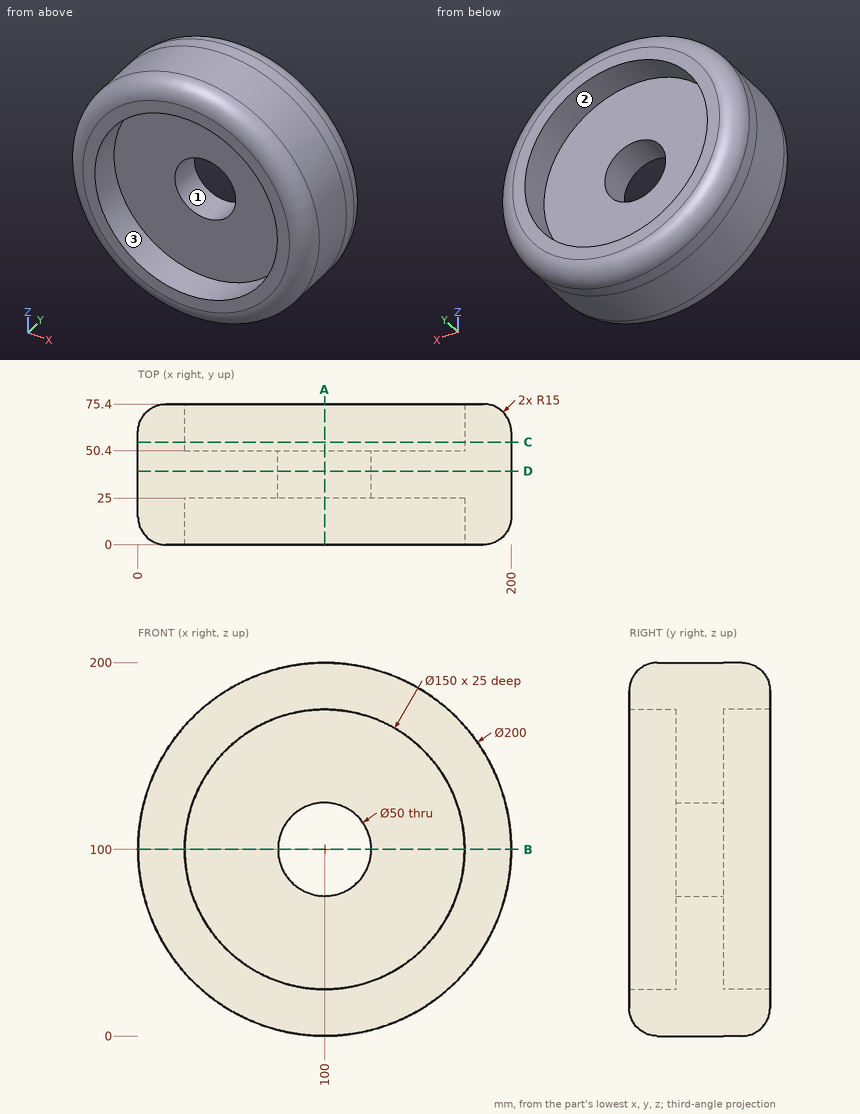
Here's the drawing with two shaded views (mm, measured from the low corner). I have some questions. A direction names the side the tool comes from. Coordinates: 2 decimals unless noted, no trailing zeros. Write each loop counter-clockwise with the first axis right and the second up, starting at its lowest first coordinate (ties: lowest second). Pieces come first, ordered by that corner, then holes. Notation, with made-up numbers: (60.25, 56) - (113.25, 56) arc R11 cw to (113.25, 68) - close; hole circle Ø2 at (-7.75, -18.75). An arc over 180 degrees is marked (long way). Return JSON: item names as keys, results as strings.
Q1. I'm going to push flat-ended pins straight in: pin 1 Ø5 at (y, z) = (29, 88) entering from -X; pin 2 Ø8 at (y, z) = (50, 27) entering from +X; pin 3 Ø12 at (y, z) = (36, 76.5) entering from +X. Where does each tip first touch, or does it pass through?
Computed values:
{"pin 1": "stops at x = 0.45", "pin 2": "stops at x = 172.38", "pin 3": "stops at x = 198.46"}
Q2. If we section it at C-C (y = 55): Please give me the cut outline in (x, z), then the cut area to 3 significant figures.
Computed values:
{"outline": "circle Ø200 at (100, 100); hole circle Ø150 at (100, 100)", "area": "13,700 mm2"}
Q3. If we section it at D-D (y = 39.5): Please give me the cut outline in (x, z), then the cut area to 3 significant figures.
Computed values:
{"outline": "circle Ø200 at (100, 100); hole circle Ø50 at (100, 100)", "area": "29,500 mm2"}
Q4. On a 3-axis mill with a long thin cutter (end or side, diameter ignored), from which of +Z, -Z, +X, -X, +Y, -Y can I reach the whole of each face in a straight line? I mean the marked faces 1, 2 and 3. Say none if no direction works.
Computed values:
{"face 1": "+Y, -Y", "face 2": "+Y", "face 3": "-Y"}
Q5. Please list where these lines run through material, in increasing order: L1, parallel to Z at x = 100, y = 16; L2, parallel to Z at x = 100, y = 38; L3, parallel to Y at x = 107, z = 151. Write a range as from..to.
Computed values:
{"L1": "z = 0..25, 175..200", "L2": "z = 0..75, 125..200", "L3": "y = 25..50.4"}
Q6. If we section it at A-A (x = 100): Please give me the cut outline in (y, z).
Computed values:
{"outline": "(0, 15) arc R15 ccw to (15, 0) - (60.4, 0) arc R15 ccw to (75.4, 15) - (75.4, 25) - (50.4, 25) - (50.4, 75) - (25, 75) - (25, 25) - (0, 25) - close; (0, 175) - (25, 175) - (25, 125) - (50.4, 125) - (50.4, 175) - (75.4, 175) - (75.4, 185) arc R15 ccw to (60.4, 200) - (15, 200) arc R15 ccw to (0, 185) - close"}
Q7. If we section it at B-B (z = 100): Please give me the cut outline in (x, y).
Computed values:
{"outline": "(0, 15) arc R15 ccw to (15, 0) - (25, 0) - (25, 25) - (75, 25) - (75, 50.4) - (25, 50.4) - (25, 75.4) - (15, 75.4) arc R15 ccw to (0, 60.4) - close; (125, 25) - (175, 25) - (175, 0) - (185, 0) arc R15 ccw to (200, 15) - (200, 60.4) arc R15 ccw to (185, 75.4) - (175, 75.4) - (175, 50.4) - (125, 50.4) - close"}
